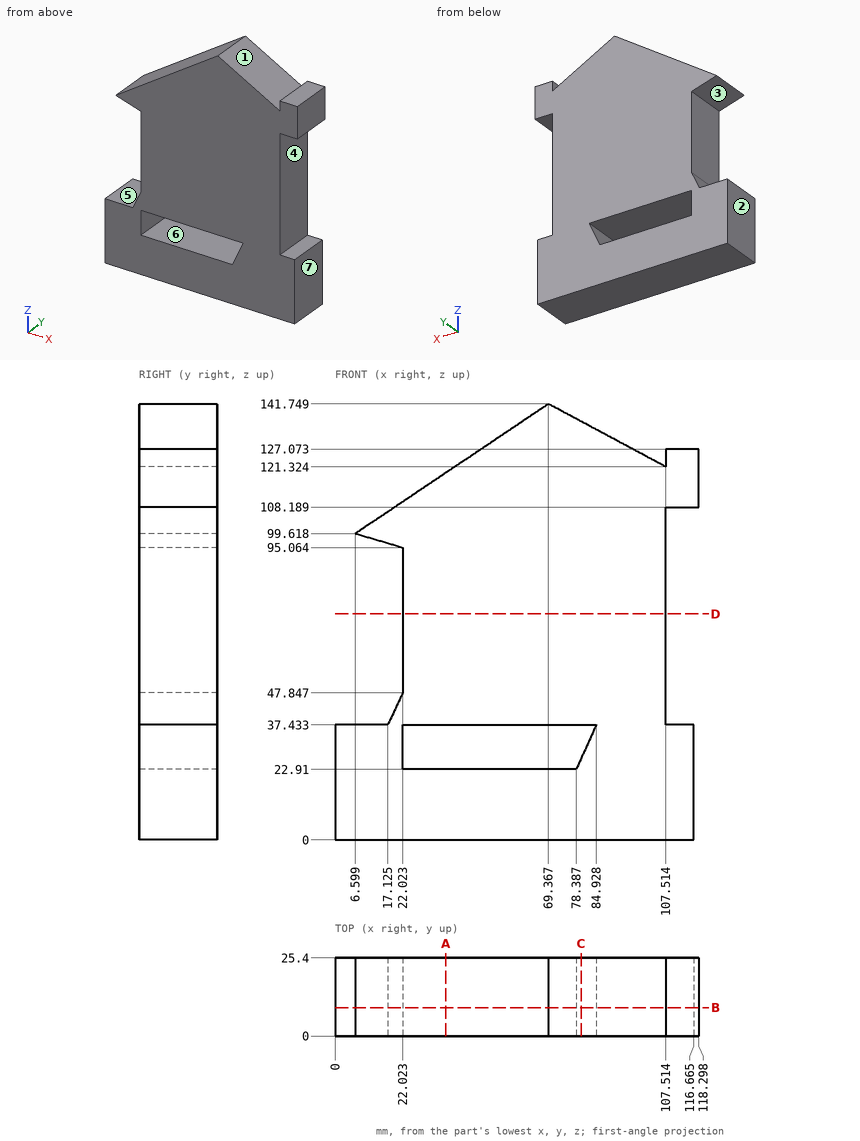
The figure shows three views and two pictorial views of one solid part (mm, origin at its lowest corner). Answer the questions. A direction names the side the tool comes from. Coordinates: 2 decimals unless noted, no trailing zeros. Write each loop counter-clockwise with the first axis right and the second up, starting at its lowest first coordinate (ties: lowest second). Pieces come first, ordered by that corner, then holes.
1. For the marked faces 5, 6 and 7, determine the directions among +Z, -Z, +X, -X, +Y, -Y from which every point of the face is accessible in a straight line to the end or side of a thin tool.
Results list:
face 5: -X, +Y, -Y
face 6: +Y, -Y
face 7: -Z, +X, +Y, -Y
2. For a pull along Z with two mould halves and no side action, classify the marked faces 1, 2, 3 and 4 as +Z half, -Z half, draft (parallel to the pull), parting line (faces both ways), or undercut.
Results list:
face 1: +Z half
face 2: draft
face 3: undercut
face 4: undercut
3. The part is cut by section A-A, the plane x = 36. Write down the section's boundary in (y, z), and give its area (3 significant figures).
Results list:
outline: (0, 0) - (25.4, 0) - (25.4, 22.91) - (0, 22.91) - close; (0, 37.43) - (25.4, 37.43) - (25.4, 119.35) - (0, 119.35) - close
area: 2,660 mm2
4. Flat-ended cylindrical pins translate along their axes: pin 1 (4 mm diameter, centred on y = 11, z = 31, fed in from +X) (1 decimal); pin 2 (4 mm diameter, centred on y = 21.5, z = 112.5, fed in from -X); pin 3 (4 mm diameter, centred on y = 10.5, z = 89.5, fed in from +X). Find the tip coordinate at first contact, or state that the pin passes through.
Results list:
pin 1: stops at x = 116.7
pin 2: stops at x = 22.81
pin 3: stops at x = 107.51
5. The part is cut by section D-D, the plane z = 73.5. Write down the section's boundary in (x, y).
Results list:
outline: (22.02, 0) - (107.51, 0) - (107.51, 25.4) - (22.02, 25.4) - close
6. The part is cut by section B-B, the plane y = 9.25. Write down the section's boundary in (x, z) (1 decimal).
Results list:
outline: (0, 0) - (116.7, 0) - (116.7, 37.4) - (107.5, 37.4) - (107.5, 108.2) - (118.3, 108.2) - (118.3, 127.1) - (107.5, 127.1) - (107.5, 121.3) - (69.4, 141.7) - (6.6, 99.6) - (22, 95.1) - (22, 47.8) - (17.1, 37.4) - (0, 37.4) - close; hole (22, 22.9) - (78.4, 22.9) - (84.9, 37.4) - (22, 37.4) - close
7. The part is cut by section C-C, the plane x = 80. Write down the section's boundary in (y, z) (1 decimal), and give its area (3 significant figures).
Results list:
outline: (0, 0) - (25.4, 0) - (25.4, 26.5) - (0, 26.5) - close; (0, 37.4) - (25.4, 37.4) - (25.4, 136.1) - (0, 136.1) - close
area: 3,180 mm2
8. Consider line 1 along Z through (x, y) = (109, 18.5); line 2 along Z through (x, y) = (32, 14) (1 decimal); line 3 along X through (y, z) = (7.5, 80.5). Determine where each line is inside the solid, lowest interval first.
Results list:
line 1: z = 0 to 37.43, 108.19 to 127.07
line 2: z = 0 to 22.9, 37.4 to 116.7
line 3: x = 22.02 to 107.51
